```python
from build123d import *

# Parameters (mm, degrees)
SKETCH1_W                      = 339.85
SKETCH1_H                      = 40
BOSS_EXTRUDE1_DEPTH            = 40
SKETCH2_W                      = 34
SKETCH2_H                      = 34
CUT_EXTRUDE1_DEPTH             = 395.033022093
F_5_6_5_6_DIAMETER_HOLE1_D     = 5.6
F_5_6_5_6_DIAMETER_HOLE1_DEPTH = 3
F_5_6_5_6_DIAMETER_HOLE2_D     = 5.6
F_5_6_5_6_DIAMETER_HOLE2_DEPTH = 3
F_5_6_5_6_DIAMETER_HOLE3_D     = 5.6
F_5_6_5_6_DIAMETER_HOLE4_D     = 5.6
F_5_6_5_6_DIAMETER_HOLE4_DEPTH = 40
CHAMFER1_SIZE                  = 0.5


with BuildPart() as part:
    # Sketch1 → Boss-Extrude1 (new body)
    with BuildSketch(Plane(origin=(0, -102, 0), x_dir=(1, 0, 0), z_dir=(0, 1, 0))):
        with Locations((80.075, -120)):
            Rectangle(SKETCH1_W, SKETCH1_H)
    extrude(amount=-BOSS_EXTRUDE1_DEPTH)

    # Sketch2 → Cut-Extrude1 (cut, through all)
    with BuildSketch(Plane.ZY.offset(89.85)):
        with Locations((120, -122)):
            Rectangle(SKETCH2_W, SKETCH2_H)
    extrude(amount=-CUT_EXTRUDE1_DEPTH, mode=Mode.SUBTRACT)

    # Ø5.6 (5.6) Diameter Hole1
    with Locations(Plane(origin=(0, -139, 0), x_dir=(1, 0, 0), z_dir=(0, 1, 0))):
        with Locations((220, -130), (95, -130), (220, -110), (95, -110), (-30, -130), (-50, -130), (-30, -110)):
            Hole(F_5_6_5_6_DIAMETER_HOLE1_D / 2, depth=F_5_6_5_6_DIAMETER_HOLE1_DEPTH)

    # Ø5.6 (5.6) Diameter Hole2
    with Locations(Plane(origin=(0, 0, 100), x_dir=(-1, 0, 0), z_dir=(0, 0, -1))):
        with Locations((-190, -122), (-100, -122)):
            Hole(F_5_6_5_6_DIAMETER_HOLE2_D / 2, depth=F_5_6_5_6_DIAMETER_HOLE2_DEPTH)

    # Ø5.6 (5.6) Diameter Hole3 (through all)
    with Locations(Plane(origin=(0, 0, 137), x_dir=(-1, 0, 0), z_dir=(0, 0, -1))):
        with Locations((-190, -122), (-100, -122)):
            Hole(F_5_6_5_6_DIAMETER_HOLE3_D / 2)

    # Ø5.6 (5.6) Diameter Hole4
    with Locations(Plane(origin=(0, -102, 0), x_dir=(1, 0, 0), z_dir=(0, 1, 0))):
        with Locations((220, -130), (95, -130), (220, -110), (95, -110), (-30, -130), (-50, -130), (-30, -110)):
            Hole(F_5_6_5_6_DIAMETER_HOLE4_D / 2, depth=F_5_6_5_6_DIAMETER_HOLE4_DEPTH)

    # Chamfer1
    chamfer1_edges = [part.edges().sort_by_distance(p)[0] for p in [
        (80.075, -142, 100),
        (80.075, -139, 103),
        (80.075, -105, 103),
        (80.075, -105, 137),
        (80.075, -139, 137),
        (80.075, -142, 140),
        (80.075, -102, 100),
        (80.075, -102, 140),
    ]]
    chamfer(chamfer1_edges, length=CHAMFER1_SIZE)


solid = part.part
```
The listing builds one solid part. Answer for the finished solid, in the listing's coordinates (mm). A direction names the side the tool comes from. Give positions to 0.01 mm unless a question says otherwise; leave off trailing zeros. Loops run counter-clockwise (first coordinate to the right, second up) from the corner with the lowest first, then second, coordinate; pieces in that order, holes last. Notation, with made-up numbers: (3, 75) - (59, 75) arc R29 cw to (59, 105) - close; hole circle Ø1 at (70.25, -31). An arc over 180 degrees is marked (long way). Answer as CSV lines item,"result". Start each with the question number.
Item 1: The mould has two halves that part along Y. Classify faces 1 (the face through (78, -122, 100)), 2 (the face through (78, -105, 120)), 3 (the face through (78, -142, 120)): +Y half, -Y half, draft (parallel to the pull), parting line (faces both ways), or undercut.
Item 2: For faces 4 (the face through (78, -122, 103)), 5 (the face through (-29.635, -140.521, 107.224)), determine the directions among +Z, -Z, +X, -X, +Y, -Y from which every point of the face is accessible in a straight line to the end or side of a thin tool.
Item 3: A cutting plane is placed at B-B on z = 119. Determine the outline of the cut face in (x, y), then the cut area to 3 significant figures.
Item 4: This flat-tipped pin is pushed along its axis until it touches: pin 1 (5 mm diameter, centred on x = 220, z = 110, fed in from -Y). Where does it stop, or does it pass through?
Item 5: Find the intervals of material crossed by line 1 (Z direction, x = 95, y = -140.65); line 2 (X direction, y = -140.5, z = 110); line 3 (X direction, y = -104, z = 130), in increasing order. Write a range as from..to.
Item 6: A cutting plane is placed at A-A on y = -134. Determine the outline of the cut face in (x, z), then the cut area to 3 significant figures.
Item 7: A cutting plane is placed at C-C on x = 220. Count the separate pieces of the cut face and the enclosed holes in it, then the cut area to 3 significant figures.
Found:
1,face 1,"draft"
1,face 2,"undercut"
1,face 3,"-Y half"
2,face 4,"+X, -X"
2,face 5,"+Y, -Y"
3,outline,"(-89.85, -142) - (250, -142) - (250, -139) - (-89.85, -139) - close; (-89.85, -105) - (250, -105) - (250, -102) - (-89.85, -102) - close"
3,area,"2,040 mm^2"
4,pin 1,"passes through"
5,line 1,"z = 100..107.2, 112.8..127.2, 132.8..140"
5,line 2,"x = -89.85..-32.8, -27.2..92.2, 97.8..217.2, 222.8..250"
5,line 3,"x = -89.85..-52.8, -47.2..-32.8, -27.2..92.2, 97.8..217.2, 222.8..250"
6,outline,"(-89.85, 100) - (250, 100) - (250, 103) - (-89.85, 103) - close; (-89.85, 137) - (250, 137) - (250, 140) - (-89.85, 140) - close"
6,area,"2,040 mm^2"
7,separate pieces,"4"
7,enclosed holes,"0"
7,area,"377 mm^2"
